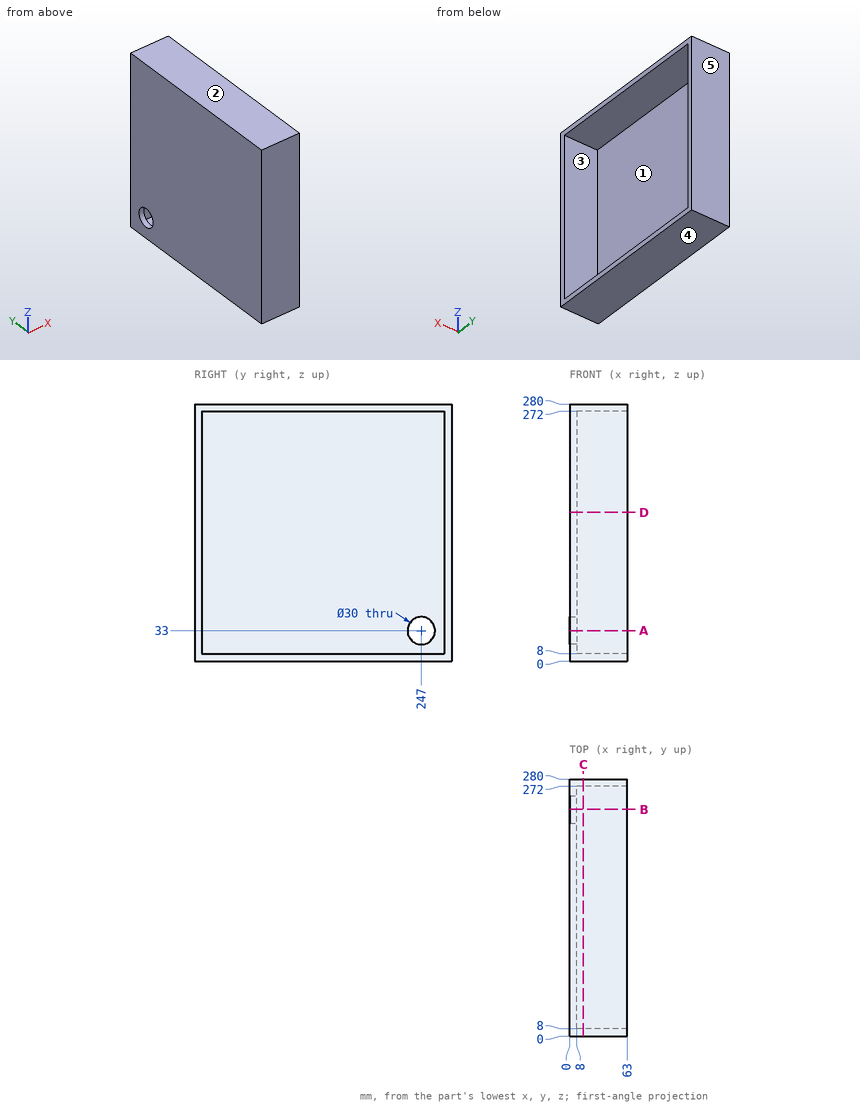
Geometry check sheet. Reference: drawing and pictorial views, mm from the part's lowest x, y, z. A direction names the side the tool comes from. Give positions to 0.01 mm unless a question says otherwise; leave off trailing zeros. Write each loop counter-clockwise with the first axis right and the second up, starting at its lowest first coordinate (ties: lowest second). Pieces come first, ordered by that corner, then holes.
Item 1: Scan lines: L1, parallel to Z at x = 10.5, y = 117; L2, parallel to Y at x = 4.5, z = 33. Record each from-to range of solid material in increasing order.
Item 2: Gauge pin test, flat ends, axial feed: pin 1 (4 mm diameter, centred on y = 191, z = 144.5, fed in from +X); pin 2 (3 mm diameter, centred on x = 52.5, y = 143, fed in from -Z); pin 3 (18 mm diameter, centred on y = 247, z = 33, fed in from +X). Record the tip position at first contact, or that the pin passes through.
Item 3: Draft check along Y on the marked faces 3, 4 and 5. Enter one of: released by +Y, released by -Y, zero draft, split by the parting line, or undercut.
Item 4: Cross-section at B-B (y = 247). Enter the section's corners in (x, z).
Item 5: Cross-section at A-A (z = 33). Enter the section's corners in (x, y).
Item 6: Access from +Z, -Z, +X, -X, +Y, -Y to the whole of each face (thin tool, end or side, straight path). Record for the marked faces 1 and 2.
Item 7: Cross-section at C-C (x = 15). Enter the section's corners in (y, z), and give its area (3 significant figures).
Item 8: Cross-section at D-D (z = 162). Enter the section's corners in (x, y).
Report:
1. L1: z = 0 to 8, 272 to 280
1. L2: y = 0 to 232, 262 to 280
2. pin 1: stops at x = 8
2. pin 2: stops at z = 0
2. pin 3: passes through
3. face 3: undercut
3. face 4: zero draft
3. face 5: released by +Y
4. outline: (0, 0) - (63, 0) - (63, 8) - (8, 8) - (8, 18) - (0, 18) - close; (0, 48) - (8, 48) - (8, 272) - (63, 272) - (63, 280) - (0, 280) - close
5. outline: (0, 0) - (63, 0) - (63, 8) - (8, 8) - (8, 232) - (0, 232) - close; (0, 262) - (8, 262) - (8, 272) - (63, 272) - (63, 280) - (0, 280) - close
6. face 1: +X
6. face 2: +Z, +X, -X, +Y, -Y
7. outline: (0, 0) - (280, 0) - (280, 280) - (0, 280) - close; hole (8, 8) - (272, 8) - (272, 272) - (8, 272) - close
7. area: 8,700 mm2
8. outline: (0, 0) - (63, 0) - (63, 8) - (8, 8) - (8, 272) - (63, 272) - (63, 280) - (0, 280) - close
